Could you check a few things on this model? Use its own coordinates, in mm. A direction names the side the tool comes from. Round coordinates to 2 decimals unless told otherwise and drop trailing zeros. Loops run counter-clockwise (first coordinate to the right, second up) from the corner with the lowest first, then second, coordinate; pieces in that order, holes last. Notation, with made-up numbers: M 59,-31 L 66,-31 A26 cw 66,1 Z; hole C 44.5,32.5 d6. An arc over 180 degrees is marked long. Return JSON: item names as keys, results as strings. Group by question number.
```python
from build123d import *

# Parameters (mm, degrees)
SKETCH1_W                                 = 181.991
SKETCH1_H                                 = 118.999
BOSS_EXTRUDE1_DEPTH                       = 203.2
SKETCH2_W                                 = 141.3002
SKETCH2_H                                 = 141.3002
BOSS_EXTRUDE2_DEPTH                       = 16.8021
SKETCH3_R                                 = 14.2875
BOSS_EXTRUDE3_DEPTH                       = 66.7004
TAP_DRILL_FOR_3_8_16_TAP1_D               = 7.9375
TAP_DRILL_FOR_3_8_16_TAP1_DEPTH           = 12.7
TAP_DRILL_FOR_3_8_16_TAP1_TIP             = 2.384665582
TAP_DRILL_FOR_3_8_16_TAP1_ON_FACE_2_D     = 7.9375
TAP_DRILL_FOR_3_8_16_TAP1_ON_FACE_2_DEPTH = 12.7
TAP_DRILL_FOR_3_8_16_TAP1_ON_FACE_2_TIP   = 2.384665582
CHAMFER1_SIZE                             = 10.033
SKETCH7_R                                 = 57.15
BOSS_EXTRUDE4_DEPTH                       = 37.5031
SKETCH8_R                                 = 82.4992
BOSS_EXTRUDE5_DEPTH                       = 7.9756


with BuildPart() as part:
    # Sketch1 → Boss-Extrude1 (new body)
    with BuildSketch(Plane(origin=(0, 0, 0), x_dir=(1, 0, 0), z_dir=(0, 1, 0))):
        Rectangle(SKETCH1_W, SKETCH1_H)
    extrude(amount=BOSS_EXTRUDE1_DEPTH)

    # Sketch2 → Boss-Extrude2 (add)
    with BuildSketch(Plane.XY.offset(59.4995)):
        with Locations((0, 70.6501)):
            Rectangle(SKETCH2_W, SKETCH2_H)
    boss_extrude2 = extrude(amount=BOSS_EXTRUDE2_DEPTH)

    # Sketch3 → Boss-Extrude3 (add)
    with BuildSketch(Plane.XY.offset(76.3016)):
        with Locations(Location((0, 70.6501, 0), (0, 0, 180))):
            Circle(SKETCH3_R)
    extrude(amount=BOSS_EXTRUDE3_DEPTH)

    # Tap Drill for 3/8-16 Tap1
    with Locations(Plane(origin=(-80.9625, 0, -42.8625), x_dir=(0, 0, -1), z_dir=(0, -1, 0))):
        with Locations((0, 0), (-85.725, 0), (-85.725, 161.925), (0, 161.925)):
            Hole(TAP_DRILL_FOR_3_8_16_TAP1_D / 2, depth=TAP_DRILL_FOR_3_8_16_TAP1_DEPTH)
            with Locations((0, 0, -(TAP_DRILL_FOR_3_8_16_TAP1_DEPTH + TAP_DRILL_FOR_3_8_16_TAP1_TIP / 2))):  # 118° drill point
                Cone(0, TAP_DRILL_FOR_3_8_16_TAP1_D / 2, TAP_DRILL_FOR_3_8_16_TAP1_TIP, mode=Mode.SUBTRACT)

    # Tap Drill for 3/8-16 Tap1 on face 2
    with Locations(Plane(origin=(80.9625, 203.2, -42.8625), x_dir=(0, 0, 1), z_dir=(0, 1, 0))):
        with Locations((0, 0), (85.725, 0), (85.725, -161.925), (0, -161.925)):
            Hole(TAP_DRILL_FOR_3_8_16_TAP1_ON_FACE_2_D / 2, depth=TAP_DRILL_FOR_3_8_16_TAP1_ON_FACE_2_DEPTH)
            with Locations((0, 0, -(TAP_DRILL_FOR_3_8_16_TAP1_ON_FACE_2_DEPTH + TAP_DRILL_FOR_3_8_16_TAP1_ON_FACE_2_TIP / 2))):  # 118° drill point
                Cone(0, TAP_DRILL_FOR_3_8_16_TAP1_ON_FACE_2_D / 2, TAP_DRILL_FOR_3_8_16_TAP1_ON_FACE_2_TIP, mode=Mode.SUBTRACT)

    # Chamfer1
    chamfer1_edges = [part.edges().sort_by_distance(p)[0] for p in [
        (90.9955, 101.6, 59.4995),
        (-90.9955, 101.6, 59.4995),
        (-90.9955, 101.6, -59.4995),
        (90.9955, 101.6, -59.4995),
    ]]
    chamfer(chamfer1_edges, length=CHAMFER1_SIZE)

    # Mirror1: Boss-Extrude2 across plane
    add(boss_extrude2.mirror(Plane.XY))

    # Sketch7 → Boss-Extrude4 (add)
    with BuildSketch(Plane(origin=(90.9955, 0, 0), x_dir=(0, 0, -1), z_dir=(1, 0, 0))):
        with Locations(Location((0, 141.3002, 0), (0, 0, 149.946203095))):
            Circle(SKETCH7_R)
    extrude(amount=BOSS_EXTRUDE4_DEPTH)

    # Sketch8 → Boss-Extrude5 (add)
    with BuildSketch(Plane(origin=(128.4986, 0, 0), x_dir=(0, 0, -1), z_dir=(1, 0, 0))):
        with Locations((0, 141.3002)):
            Circle(SKETCH8_R)
    extrude(amount=-BOSS_EXTRUDE5_DEPTH)


solid = part.part
```
1. I need wall thicknesses on probe 1 along X at (y, z) = (28, -62.5); probe 2 along Z at (x, y) = (17.5, 27.5); probe 3 along Y at (x, z) = (56, 29). Which ranges of each line are inside material? Lowest first, please.
2. If we section it at C-C, the plane z = 65.5: Please give me the cut outline in (x, y), then the cut area to 3 significant figures.
3. If we section it at D-D, the plane y = 120: Please give me the cut outline in (x, z).
4. On a 3-axis mill with a long thin cutter (end or side, diameter ignored), from which of +Z, -Z, +X, -X, +Y, -Y can I reach the whole of each face in a straight line? I mean faces 4 (the face through (-70.65, 70, -68)), 5 (the face through (77.09, 6.44, 42)), 6 (the face through (124.567, 223.097, 10.74)), 7 (the face through (70.65, 70, 68)). Say none if no direction works.
5. If we section it at B-B, the plane x = 0: Please give me the cut outline in (y, z).
6. We'd pull the mould along Z, two halves only. Please class faces 1 (the face through (-81.635, 188.529, 42.713)), 2 (the face through (-1, 0, -1)), 3 (the face through (105.553, 198.393, -2.566)): +Z half, -Z half, draft (parallel to the pull), parting line (faces both ways), or undercut.
7. I'm going to push flat-ended pins straight in: pin 1 Ø3 at (y, z) = (172, -53) entering from -X; pin 2 Ø3 at (x, z) = (85, -42) entering from +Y; pin 3 Ø1 at (y, z) = (154, 79) entering from -X. Where does each tip first touch, or does it pass through?
8. If we section it at A-A, the plane z = 0: Please give me the cut outline in (x, y).
Geometry results:
{
 "1": {"probe 1": "-70.65 to 70.65", "probe 2": "-76.3 to 76.3", "probe 3": "0 to 203.2"},
 "2": {"outline": "M -70.65,0 L 70.65,0 L 70.65,141.3 L -70.65,141.3 Z; M 120.52,91.14 L 128.5,91.14 L 128.5,191.46 L 120.52,191.46 Z", "area": "20,800 mm^2"},
 "3": {"outline": "M -91,-49.47 L -80.96,-59.5 L -70.65,-59.5 L -70.65,-76.3 L 70.65,-76.3 L 70.65,-59.5 L 80.96,-59.5 L 91,-49.47 L 91,-53.03 L 120.52,-53.03 L 120.52,-79.7 L 128.5,-79.7 L 128.5,79.7 L 120.52,79.7 L 120.52,53.03 L 91,53.03 L 91,49.47 L 80.96,59.5 L 70.65,59.5 L 70.65,76.3 L -70.65,76.3 L -70.65,59.5 L -80.96,59.5 L -91,49.47 Z"},
 "4": {"face 4": "-Z, -X, +Y, -Y", "face 5": "-Y", "face 6": "+X", "face 7": "+Z, +Y, -Y"},
 "5": {"outline": "M 0,-76.3 L 141.3,-76.3 L 141.3,-59.5 L 203.2,-59.5 L 203.2,59.5 L 141.3,59.5 L 141.3,76.3 L 84.94,76.3 L 84.94,143 L 56.36,143 L 56.36,76.3 L 0,76.3 Z"},
 "6": {"face 1": "undercut", "face 2": "draft", "face 3": "parting line"},
 "7": {"pin 1": "x = -88.96", "pin 2": "y = 203.2", "pin 3": "x = 120.52"},
 "8": {"outline": "M -91,0 L 91,0 L 91,84.15 L 120.52,84.15 L 120.52,58.8 L 128.5,58.8 L 128.5,223.8 L 120.52,223.8 L 120.52,198.45 L 91,198.45 L 91,203.2 L -91,203.2 Z"}
}
